Verification items for this drawing (mm, ordinates from the low corner). Coordinates: 2 decimals unless noted, no trailing zeros. Order: outer loops, then holes, each group sorted by start corner. A loop starts at its lowest first (then second) coordinate and runs counter-clockwise, first axis right, second up. Notation, with made-up numbers: (31.5, -18) -> (43.5, -18) arc R17 cw to (43.5, -5) -> close; hole circle Ø8 at (-35, 59). An arc over 180 degrees is marked (long way). Put each result on its own line as item: value. Start each with the question number.
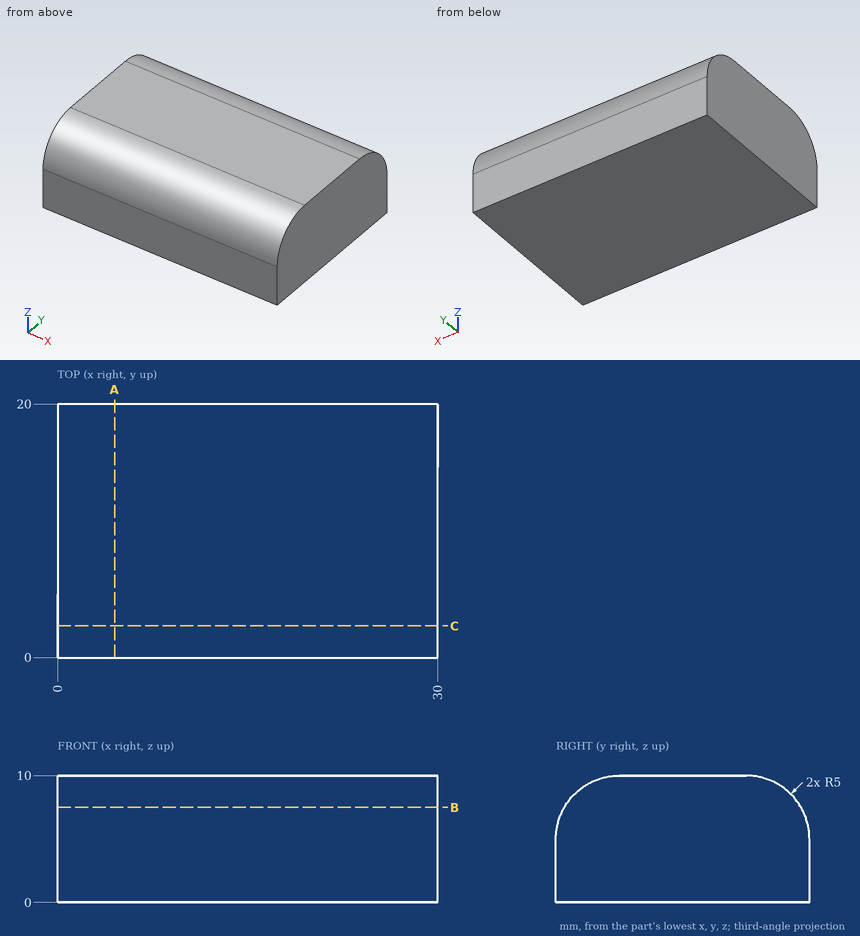
1) Sectioned sample at C-C (y = 2.5). Record the boundary of the cut face in (x, z).
2) Sectioned sample at A-A (x = 4.5). Record the boundary of the cut face in (y, z).
3) Sectioned sample at B-B (z = 7.5). Record the boundary of the cut face in (x, y).
4) Gauge pin test, flat end, axial feed: pin 1 (5 mm diameter, centred on x = 8.5, z = 8.5, fed in from +Y). Record the tip position at first contact, or that the pin passes through.
5) Scan lines: line 1 along Z through (x, y) = (24, 4); line 2 along Z through (x, y) = (23.25, 16.75); line 3 along Y through (x, z) = (19.5, 7). Record each from-to range of solid material in increasing order. Write a range as [from, to].
Entries:
1. outline: (0, 0) -> (30, 0) -> (30, 9.33) -> (0, 9.33) -> close
2. outline: (0, 0) -> (20, 0) -> (20, 5) arc R5 ccw to (15, 10) -> (5, 10) arc R5 ccw to (0, 5) -> close
3. outline: (0, 0.67) -> (30, 0.67) -> (30, 19.33) -> (0, 19.33) -> close
4. pin 1: stops at y = 19.9
5. line 1: z = [0, 9.9]
5. line 2: z = [0, 9.68]
5. line 3: y = [0.42, 19.58]
